For this review, use the dimensioned drawing (mm, ordinates from the lowest corner) and the shaded views. Round coordinates to 2 decimals unless told otherwise and drop trailing zeros. Write each loop counter-clockwise with the first axis right and the second up, starting at its lowest first coordinate (ties: lowest second). Pieces come first, ordered by that corner, then holes. Notation, with made-up numbers: (40.25, 88.5) -> (96.25, 88.5) arc R31 cw to (96.25, 115.5) -> close; hole circle Ø7 at (32, 11). An arc over 180 degrees is marked (long way). Answer as CSV lines item,"result". Start each with the question number.
Item 1: For pin 1 Ø1.5 at (x, z) = (4.5, 23) entering from +Y; pin 2 Ø2.5 at (y, z) = (1, 23.5) entering from +X; pin 3 Ø1.3 at (x, z) = (5.5, 16.5) entering from +Y (3 decimals); pin 4 Ø1 at (y, z) = (94, 26.5) entering from -X, all flat-tipped, find the tip position at first contact; note any pin that passes through.
Item 2: Take a section at C-C on y = 52.5. Give the boundary of the cut face in (x, z), then the cut area to 3 significant figures.
Item 3: Mouldability with a two-part tool opening along Z and no side actions: class the marked faces 1 and 2 as +Z half, -Z half, draft (parallel to the pull), parting line (faces both ways), or undercut.
Item 4: Wall thickness on probe 1 along Z at (x, y) = (3.75, 36.5); probe 2 along Y at (x, z) = (3, 14.5); probe 3 along Z at (x, y) = (3.75, 46): over which ranges is each line inside the solid? List them lowest first. Write a range as from..to.
Item 5: Take a section at B-B on x = 2.5. Give the boundary of the cut face in (y, z), then the cut area to 3 significant figures.
Item 6: Take a section at D-D on z = 11.5. Give the boundary of the cut face in (x, y) (3 decimals), then the cut area to 3 significant figures.
Item 7: Take a section at A-A on z = 30. Give the boundary of the cut face in (x, y) (3 decimals), then the cut area to 3 significant figures.
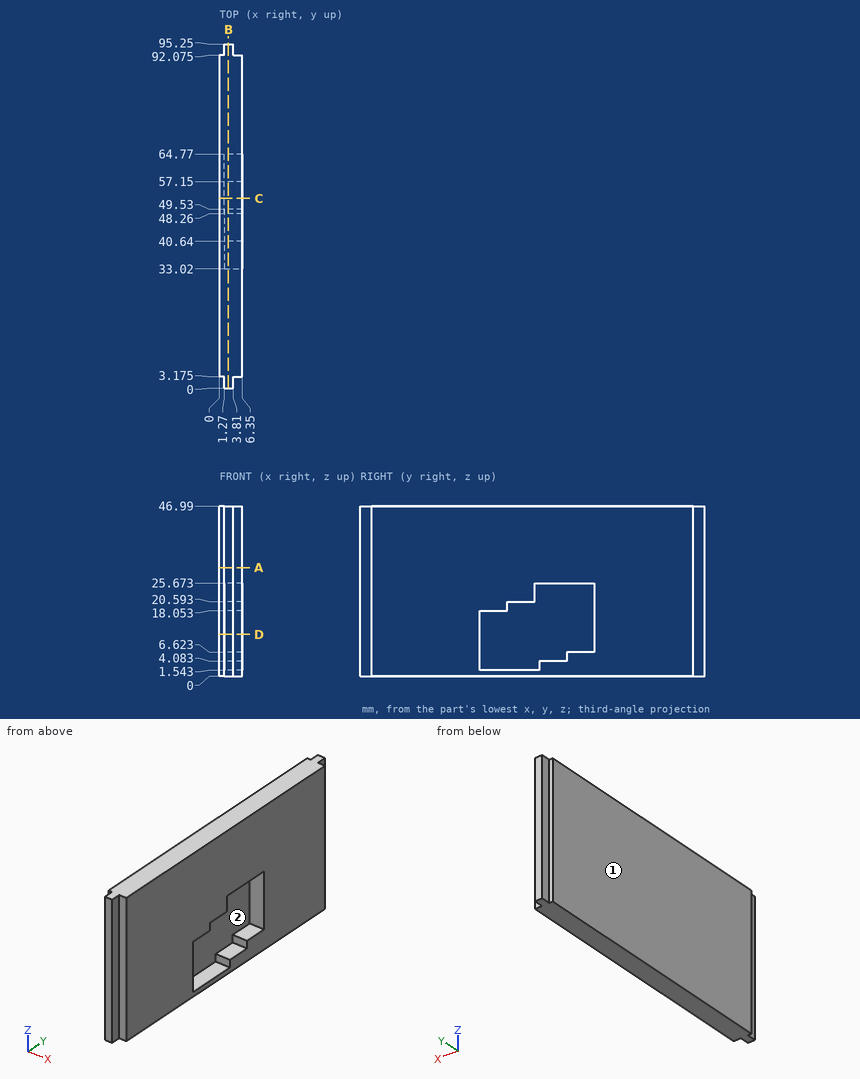
Output values:
1,pin 1,"stops at y = 95.25"
1,pin 2,"stops at x = 3.81"
1,pin 3,"stops at y = 92.075"
1,pin 4,"stops at x = 1.27"
2,outline,"(0, 0) -> (6.35, 0) -> (6.35, 4.08) -> (1.27, 4.08) -> (1.27, 25.67) -> (6.35, 25.67) -> (6.35, 46.99) -> (0, 46.99) -> close"
2,area,"189 mm^2"
3,face 1,"draft"
3,face 2,"undercut"
4,probe 1,"z = 0..1.54, 18.05..46.99"
4,probe 2,"y = 0..33.02, 64.77..95.25"
4,probe 3,"z = 0..1.54, 20.59..46.99"
5,outline,"(0, 0) -> (95.25, 0) -> (95.25, 46.99) -> (0, 46.99) -> close; hole (33.02, 1.54) -> (49.53, 1.54) -> (49.53, 4.08) -> (57.15, 4.08) -> (57.15, 6.62) -> (64.77, 6.62) -> (64.77, 25.67) -> (48.26, 25.67) -> (48.26, 20.59) -> (40.64, 20.59) -> (40.64, 18.05) -> (33.02, 18.05) -> close"
5,area,"3,860 mm^2"
6,outline,"(0, 3.175) -> (1.27, 3.175) -> (1.27, 0) -> (3.81, 0) -> (3.81, 3.175) -> (6.35, 3.175) -> (6.35, 33.02) -> (1.27, 33.02) -> (1.27, 64.77) -> (6.35, 64.77) -> (6.35, 92.075) -> (3.81, 92.075) -> (3.81, 95.25) -> (1.27, 95.25) -> (1.27, 92.075) -> (0, 92.075) -> close"
6,area,"419 mm^2"
7,outline,"(0, 3.175) -> (1.27, 3.175) -> (1.27, 0) -> (3.81, 0) -> (3.81, 3.175) -> (6.35, 3.175) -> (6.35, 92.075) -> (3.81, 92.075) -> (3.81, 95.25) -> (1.27, 95.25) -> (1.27, 92.075) -> (0, 92.075) -> close"
7,area,"581 mm^2"
